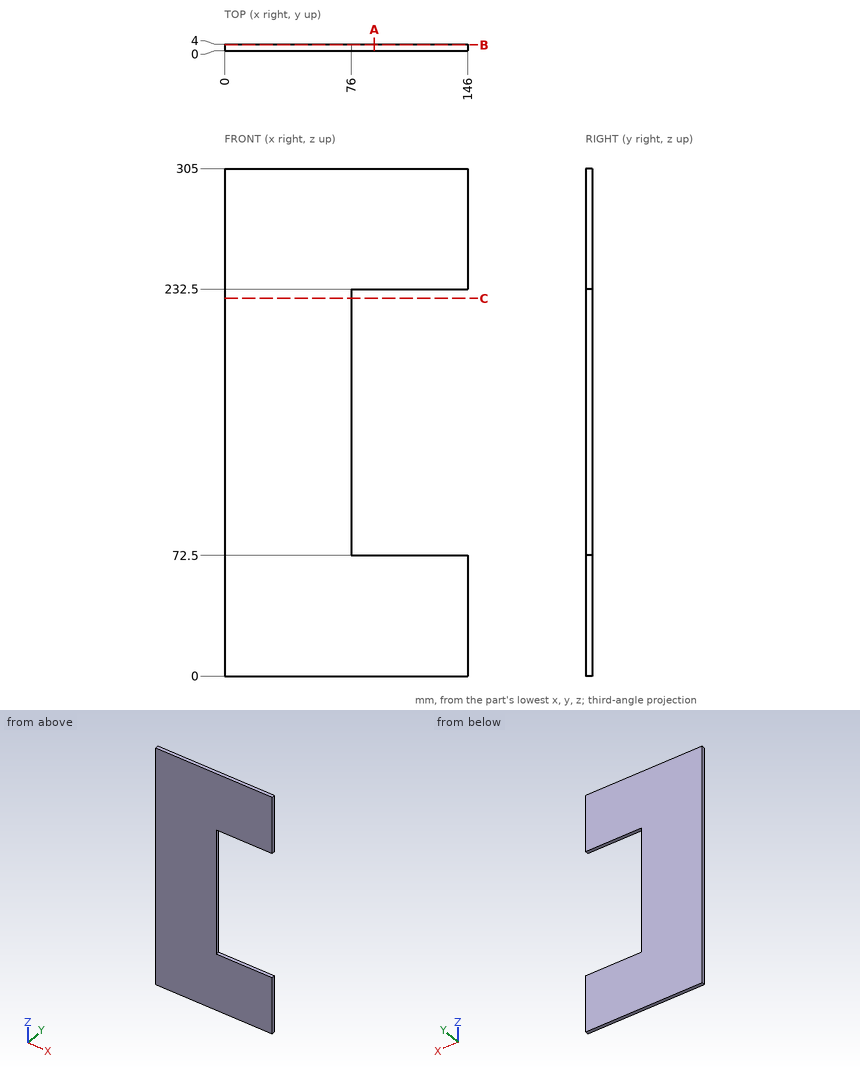
Could you check a few things on this drawing? It's one solid part, dimensions in mm from its lowest x, y, z. Coordinates: 2 decimals unless noted, no trailing zeros. Order: outer loops, then holes, each group sorted by start corner. A loop starts at its lowest first (then second) coordinate and runs counter-clockwise, first axis right, second up. Notation, with made-up numbers: M -5,-26 L 52,-26 A20 cw 52,3 Z; hole C -20,80 d8. An arc over 180 degrees is marked long. Answer as a JSON object with one key per item and string values. Group by question number.
(1) For pin 1 (1.2 mm diameter, centred on y = 3, z = 159.5, fed in from +X), with a flat end and sliding along its axis, tell me the tip position at first contact or that it passes through.
(2) Suppose I cut it at C-C, the plane z = 227. Please give me the cut outline in (x, y), then the cut area to 3 significant figures.
(3) Suppose I cut it at B-B, the plane y = 3.4. Please give me the cut outline in (x, z), then the cut area to 3 significant figures.
(4) I need wall thicknesses on probe 1 along Z at (x, y) = (118, 2.1); probe 2 along X at (y, z) = (1.8, 103). Which ranges of each line are inside material? Lowest first, please.
(5) Suppose I cut it at A-A, the plane x = 90. Please give me the cut outline in (y, z).
Values found:
{
 "1": {"pin 1": "stops at x = 76"},
 "2": {"outline": "M 0,0 L 76,0 L 76,4 L 0,4 Z", "area": "304 mm^2"},
 "3": {"outline": "M 0,0 L 146,0 L 146,72.5 L 76,72.5 L 76,232.5 L 146,232.5 L 146,305 L 0,305 Z", "area": "33,300 mm^2"},
 "4": {"probe 1": "z = 0 to 72.5, 232.5 to 305", "probe 2": "x = 0 to 76"},
 "5": {"outline": "M 0,0 L 4,0 L 4,72.5 L 0,72.5 Z; M 0,232.5 L 4,232.5 L 4,305 L 0,305 Z"}
}
